```python
from build123d import *

# Parameters (mm, degrees)
BOX_W                             = 70
BOX_H                             = 200
BOX_DEPTH                         = 11.6
POCKET_DEPTH                      = 200.001
LINEARPATTERN_COUNT               = 5
LINEARPATTERN_PITCH               = 14.5
SKETCH_W                          = 82.408782
SKETCH_H                          = 38.885188
SKETCH_W_2                        = 6
SKETCH_H_2                        = 21.094656
POCKET001_DEPTH                   = 200.001
SKETCH003_R                       = 1
POCKET002_DEPTH                   = 5.201
SKETCH004_R                       = 1
POCKET003_DEPTH                   = 15
SKETCH005_R                       = 2
POCKET004_DEPTH                   = 4.5
FILLET_R                          = 1.1
PART_MIRRORING001_PLACEMENT_ANGLE = 180


with BuildPart() as fillet_body:
    # Box → Box (new body)
    with BuildSketch(Plane(origin=(-7.5, 0, 0), x_dir=(1, 0, 0), z_dir=(0, 0, 1))):
        with Locations((35, 100)):
            Rectangle(BOX_W, BOX_H)
    extrude(amount=BOX_DEPTH)

    # Sketch002 → Pocket (cut, through all)
    with BuildSketch(Plane(origin=(-7.5, 0, 0), x_dir=(1, 0, 0), z_dir=(0, -1, 0))):
        Polygon((14.1, 10), (11.2, 10), (11.2, 3), (2.7, 3), (2.7, 10), (1.9, 10), (1.9, 10.4), (2.25, 11.6), (13.75, 11.6), (14.1, 10.4), align=None)
    pocket = extrude(amount=-POCKET_DEPTH, mode=Mode.SUBTRACT)

    # LinearPattern: Pocket ×5
    with Locations(*[(i * LINEARPATTERN_PITCH, 0, 0) for i in range(1, LINEARPATTERN_COUNT)]):
        add(pocket, mode=Mode.SUBTRACT)

    # Sketch → Pocket001 (cut, through all)
    with BuildSketch(Plane(origin=(-7.5, 0, 0), x_dir=(1, 0, 0), z_dir=(0, -1, 0))):
        with Locations((35.413628, 6.289411)):
            Rectangle(SKETCH_W, SKETCH_H)
        with Locations((14.2, 4.644143)):
            Rectangle(SKETCH_W_2, SKETCH_H_2, mode=Mode.SUBTRACT)
    extrude(amount=-POCKET001_DEPTH, mode=Mode.SUBTRACT)

    # Sketch003 → Pocket002 (cut, through all)
    with BuildSketch(Plane.YZ.offset(8.9)):
        with Locations((21.45, -100)):
            Circle(SKETCH003_R)
        with Locations((21.45, -10)):
            Circle(SKETCH003_R)
        with Locations((21.45, -190)):
            Circle(SKETCH003_R)
    extrude(amount=-POCKET002_DEPTH, mode=Mode.SUBTRACT)

    # Sketch004 → Pocket003 (cut)
    with BuildSketch(Plane(origin=(-7.5, 0, 0), x_dir=(1, 0, 0), z_dir=(0, 0, -1))):
        with Locations((14.2, -190)):
            Circle(SKETCH004_R)
        with Locations((14.2, -100)):
            Circle(SKETCH004_R)
        with Locations((14.2, -10)):
            Circle(SKETCH004_R)
    extrude(amount=-POCKET003_DEPTH, mode=Mode.SUBTRACT)

    # Sketch005 → Pocket004 (cut)
    with BuildSketch(Plane(origin=(-7.5, 0, 11.6), x_dir=(1, 0, 0), z_dir=(0, 0, 1))):
        with Locations((14.2, 190)):
            Circle(SKETCH005_R)
        with Locations((14.2, 100)):
            Circle(SKETCH005_R)
        with Locations((14.2, 10)):
            Circle(SKETCH005_R)
    extrude(amount=-POCKET004_DEPTH, mode=Mode.SUBTRACT)

    # Fillet
    fillet_edges = [fillet_body.edges().sort_by_distance(p)[0] for p in [
        (5.15, 0, 10),
        (6.6, 0, 10.2),
        (6.425, 0, 11),
        (9.3, 0, 10),
        (8.9, 0, 10.2),
        (9.075, 0, 11),
        (5.15, 200, 10),
        (6.6, 200, 10.2),
        (6.425, 200, 11),
        (9.075, 200, 11),
        (8.9, 200, 10.2),
        (9.3, 200, 10),
    ]]
    fillet(fillet_edges, radius=FILLET_R)


with BuildPart() as part_mirroring001:
    # Part__Mirroring001: instance of Fillet body
    add(fillet_body.part.mirror(Plane(origin=(0, 0, 0), x_dir=(0, -1, 0), z_dir=(1, 0, 0))))


with BuildPart() as part_mirroring001_1:
    # Part__Mirroring001 placement: moved
    add(part_mirroring001.part.moved(Location((14.5, 200, 0))).rotate(Axis((14.5, 200, 0), (0, 0, 1)), PART_MIRRORING001_PLACEMENT_ANGLE))


solid = part_mirroring001_1.part
```
Part model, mm, in its own coordinate system. A direction names the side the tool comes from. Round coordinates to 2 decimals unless told otherwise and drop trailing zeros. Loops run counter-clockwise (first coordinate to the right, second up) from the corner with the lowest first, then second, coordinate; pieces in that order, holes last. Notation, with made-up numbers: (18, 59.5) -> (61, 59.5) arc R5 cw to (61, 68.5) -> close; hole circle Ø9 at (53, 43.25). An arc over 180 degrees is marked (long way). Use CSV: the item, a comma, the result in double quotes. Start each with the question number.
1) Drop a flat-ended pin along its axis: P1, Ø2, axis at x = 22, y = 100, coming from the +Z side. Give the stop position or say it passes through.
2) Which spindle directions (+Z, -Z, +X, -X, +Y, -Y) get a long thin tool onto all of the face, cutting with end or side? Do faces 4 (the flat face through (21.2, 98.6, 0)), 5 (the flat face through (20, 190, 7.1)). Say none if no direction does.
3) Pull direction X, two halves, no side cores. Call faces 1 (the flat face through (22, 99, 7.1)), 2 (the flat face through (21, 200, 4)), 3 (the flat face through (24.2, 101, 5)): +X half, -X half, draft (parallel to the pull), parting line (faces both ways), or undercut.
4) Cut at A-A, the plane y = 70. Write the cut outline in (x, z), plus the area to 3 significant figures.
5) Wall check: L1, parallel to Y at x = 21.2, z = 5.75; L2, parallel to Y at x = 21.2, z = 8.9; L3, parallel to X at y = 10, z = 8.4. Give the ranges that are in metal, low to high. Write a range as [from, to].
Determined:
1,P1,"stops at z = 7.1"
2,face 4,"-Z, +X, -X, +Y, -Y"
2,face 5,"+Z"
3,face 1,"undercut"
3,face 2,"draft"
3,face 3,"+X half"
4,outline,"(18.2, 0) -> (24.2, 0) -> (24.2, 10) -> (23.4, 10) -> (23.4, 10.4) -> (23.75, 11.6) -> (20.75, 11.6) -> (21.1, 10.4) -> (21.1, 10) -> (18.2, 10) -> close"
4,area,"64.1 mm2"
5,L1,"y = [0, 9], [11, 99], [101, 189], [191, 200]"
5,L2,"y = [0, 8], [12, 98], [102, 188], [192, 200]"
5,L3,"x = [18.2, 19.2], [23.2, 24.2]"
